Check sheet for the modelled part. Datum: model origin and axes. Units: mm. A direction names the side the tool comes from. Give positions to 0.01 mm unless a question says otherwise; leave off trailing zeros. Order: outer loops, then holes, each group sorted by start corner. A loop starts at its lowest first (then second) coordinate and runs counter-clockwise, first axis right, second up. Notation, with made-up numbers: (88, 9) -> (120, 9) arc R24 ccw to (120, 46) -> close; hole circle Ø11 at (86.5, 1.5). An arc over 180 degrees is marked (long way). Write each question's results on one line, items separated by ' | '.
Autodesk Inventor part; units mm, degrees
ref_plane "CP_XY" through (0, 0, 0) normal (1, 0, 0) x (0, 0, -1)
ref_plane "CP_YZ" through (0, 0, 0) normal (0, 0, -1) x (0, 1, 0)
ref_plane "CP_ZX" through (0, 0, 0) normal (0, 1, 0) x (1, 0, 0)
sketch "Sketch_1" plane through (0, 0, 0) normal (0, 0, 1) x (1, 0, 0)
  line L0 (0, 0) -> (-12, 0)
  line L1 (-12, 0) -> (-12, 4.9265)
  line L2 (-12, 4.9265) -> (-10.9265, 6)
  line L3 (-10.9265, 6) -> (-1.75, 6)
  line L4 (-1.75, 6) -> (0, 4.25)
  line L5 (0, 4.25) -> (0, 0)
  line L6 (0, 0) -> (-12, 0)
revolve "Revolution1" add sketch "Sketch_1" angle 360 about axis through (0, 0, 0) along (1, 0, 0)
thread "Thread1"
sketch "Sketch_2" plane through (-12, 0, 0) normal (-1, 0, 0) x (0, 1, 0)
  line L0 (-3, -1.7321) -> (0, -3.4641)
  line L1 (0, -3.4641) -> (3, -1.7321)
  line L2 (3, -1.7321) -> (3, 1.7321)
  line L3 (3, 1.7321) -> (0, 3.4641)
  line L4 (0, 3.4641) -> (-3, 1.7321)
  line L5 (-3, 1.7321) -> (-3, -1.7321)
extrude "Extrusion1" cut sketch "Sketch_2" against normal blind 4.8
sketch "Sketch_3" plane through (0, 0, 0) normal (0, 0, 1) x (1, 0, 0)
  line L0 (-5.4679, 0) -> (-7.2, 0)
  line L1 (-7.2, 0) -> (-7.2, 3)
  line L2 (-7.2, 3) -> (-5.4679, 0)
  line L3 (-5.4679, 0) -> (-7.2, 0)
revolve "Revolution2" cut sketch "Sketch_3" angle 360 about axis through (-5.4679, 0, 0) along (1, 0, 0)
ref_plane "CP_XY" through (0, 0, 0) normal (1, 0, 0) x (0, 0, -1)
ref_plane "CP_YZ" through (0, 0, 0) normal (0, 0, -1) x (0, 1, 0)
ref_plane "CP_ZX" through (0, 0, 0) normal (0, 1, 0) x (1, 0, 0)
properties part number "SET-SCREW12-12"
1. Mould release check, pull along Y, two halves, no side actions. Record for faces 3 (the cylindrical face through (-6, -6, 0)), 4 (the flat face through (0, 0, 0)), 5 (the flat face through (-9.6, 1.5, -2.6)): +Y half, -Y half, draft (parallel to the pull), parting line (faces both ways), or undercut.
Verdict:
face 3: parting line | face 4: draft | face 5: undercut
2. Access from +Z, -Z, +X, -X, +Y, -Y to the whole of each face (thin tool, end or side, straight path). Record for faces 1 (the flat face through (-12, 3.2, 0.1)), 2 (the flat face through (-9.6, 1.5, 2.6)).
Verdict:
face 1: +Z, -Z, -X, +Y, -Y | face 2: -X
3. Section check A-A on x = -10.75. Record the cut outline in (y, z), then the cut area to 3 significant figures.
Verdict:
outline: circle Ø12 at (0, 0); hole (-3, -1.73) -> (0, -3.46) -> (3, -1.73) -> (3, 1.73) -> (0, 3.46) -> (-3, 1.73) -> close | area: 81.9 mm^2
4. Gauge pin test, flat ends, axial feed: pin 1 Ø6 at (y, z) = (-1, -2) entering from +X; pin 2 Ø1.7 at (y, z) = (0, -2) entering from -X; pin 3 Ø5 at (x, z) = (-2, -4) entering from +Y; pin 4 Ø1 at (x, y) = (-5.5, -1) entering from +Z. Record the tip position at first contact, or that the pin passes through.
Verdict:
pin 1: stops at x = 0 | pin 2: stops at x = -7.11 | pin 3: stops at y = 5.81 | pin 4: stops at z = 5.98
5. Section check B-B on x = -6.5. Record the cut outline in (y, z), then the cut area to 3 significant figures.
Verdict:
outline: circle Ø12 at (0, 0); hole circle Ø3.58 at (0, 0) | area: 103 mm^2
6. Material ranges on probe 1 along Y at (x, z) = (-8.5, -0.5); probe 2 along Y at (x, z) = (-7.5, -2); probe 3 along Z at (x, y) = (-8.75, -2.75), recorded low to high. Write a range as from..to.
Verdict:
probe 1: y = -5.98..-3, 3..5.98 | probe 2: y = -5.66..-2.54, 2.54..5.66 | probe 3: z = -5.33..-1.88, 1.88..5.33
